Work out the finished part from the listing and answer in its coordinate system (mm). Coordinates: 2 decimals unless noted, no trailing zeros. Order: outer loops, then holes, each group sorted by start corner. A loop starts at its lowest first (then second) coordinate and runs counter-clockwise, first axis right, second up. Notation, with made-up numbers: M -29.75,64 L 24.25,64 A20 ccw 24.25,71 Z; hole C 9.5,-21.5 d4. An arc over 180 degrees is marked long. Answer in a Markdown table with one row per item. Add a question column.
Item 1: A flat-ended cylindrical pin translates along its axis: pin 1 Ø5.5 at (x, z) = (-41.25, -41.25) entering from -Y. Find the tip coordinate at first contact, or state that the pin passes through.
Item 2: The part is cut by section B-B (z = 0). Write down the section's boundary in (x, y).
Item 3: Consider line 1 (X direction, y = 1, z = -40); line 2 (Z direction, x = -7.5, y = -5.75); line 3 (X direction, y = 4.75, z = 40.5). Determine where each line is inside the solid, lowest interval first. Write a range as from..to.
Item 4: The mould has two halves that part along Z. Classify faces 1 (the face through (-1, 0, 46)), 2 (the face through (-44.645, -0.098, -44.572)), 3 (the face through (-46, 0, -1)), 4 (the face through (-40.269, 0.098, 39.365)): released by +Z, released by -Z, zero draft, split by the parting line, or undercut.
Item 5: The part is cut by section A-A (x = 23). Write down the section's boundary in (y, z), then the cut area to 3 significant figures.
Item 6: The part is cut by section C-C (y = 2.75). Write down the section's boundary in (x, z) (3 decimals), then the cut area to 3 significant figures.
from build123d import *

# Parameters (mm, degrees)
F0_W     = 92
F0_H     = 92
F0_R     = 2.125
F0_R_2   = 44
F1_DEPTH = 7
F2_R     = 4.75


with BuildPart() as f1:
    # F0 (on Front) → F1 (new body, symmetric)
    with BuildSketch(Plane.XZ):
        Rectangle(F0_W, F0_H)
        with Locations((-41.25, -41.25)):
            Circle(F0_R, mode=Mode.SUBTRACT)
        with Locations((41.25, -41.25)):
            Circle(F0_R, mode=Mode.SUBTRACT)
        with Locations((-41.25, 41.25)):
            Circle(F0_R, mode=Mode.SUBTRACT)
        Circle(F0_R_2, mode=Mode.SUBTRACT)
        with Locations((41.25, 41.25)):
            Circle(F0_R, mode=Mode.SUBTRACT)
    extrude(amount=F1_DEPTH, both=True)

    # F2
    f2_edges = [f1.edges().sort_by_distance(p)[0] for p in [
        (-46, 0, 46),
        (46, 0, 46),
        (46, 0, -46),
        (-46, 0, -46),
    ]]
    fillet(f2_edges, radius=F2_R)


solid = f1.part
Reply:
| question | item | result |
|---|---|---|
| 1 | pin 1 | stops at y = -7 |
| 2 | outline | M -46,-7 L -44,-7 L -44,7 L -46,7 Z; M 44,-7 L 46,-7 L 46,7 L 44,7 Z |
| 3 | line 1 | x = -46..-42.97, -39.53..-18.33, 18.33..39.53, 42.97..46 |
| 3 | line 2 | z = -46..-43.36, 43.36..46 |
| 3 | line 3 | x = -46..-43.24, -39.26..-17.2, 17.2..39.26, 43.24..46 |
| 4 | face 1 | released by +Z |
| 4 | face 2 | released by -Z |
| 4 | face 3 | zero draft |
| 4 | face 4 | undercut |
| 5 | outline | M -7,-46 L 7,-46 L 7,-37.51 L -7,-37.51 Z; M -7,37.51 L 7,37.51 L 7,46 L -7,46 Z |
| 5 | area | 238 mm2 |
| 6 | outline | M -46,-41.25 A4.75 ccw -41.25,-46 L 41.25,-46 A4.75 ccw 46,-41.25 L 46,41.25 A4.75 ccw 41.25,46 L -41.25,46 A4.75 ccw -46,41.25 Z; hole C 0,0 d88; hole C -41.25,-41.25 d4.25; hole C -41.25,41.25 d4.25; hole C 41.25,-41.25 d4.25; hole C 41.25,41.25 d4.25 |
| 6 | area | 2,310 mm2 |
